Build history of the part. All positions in model axes, mm. Face numbers are marked on the shaded views. A direction names the side the tool comes from. Coordinates: 2 decimals unless noted, no trailing zeros. Loops run counter-clockwise (first coordinate to the right, second up) from the corner with the lowest first, then second, coordinate; pieces in that order, holes last. Notation, with made-up numbers: (-40, 29.25) - (9, 29.25) arc R16 ccw to (9, 58.25) - close; hole circle Ø9 at (-0.5, 83.5). An arc over 180 degrees is marked (long way). One line per item, written item: value.
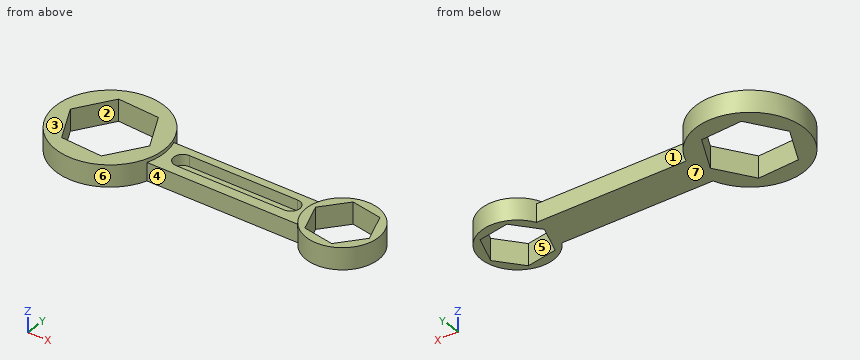
Autodesk Fusion 360 part; units mm, degrees
sketch "Sketch1" plane through (0, 0, 0) normal (0, 0, 1) x (1, 0, 0) in component "ex2"
  circle A0 centre (0, 0) radius 30
  circle A1 centre (129, 0) radius 20
  line L0 (12.7246, 19.2722) -> (-10.328, 20.6559)
  line L1 (-10.328, 20.6559) -> (-23.0525, 1.3837)
  line L2 (-23.0525, 1.3837) -> (-12.7246, -19.2722)
  line L3 (-12.7246, -19.2722) -> (10.328, -20.6559)
  line L4 (10.328, -20.6559) -> (23.0525, -1.3837)
  line L5 (23.0525, -1.3837) -> (12.7246, 19.2722)
  line L6 (146.0675, -2.9498) -> (140.0883, 13.306)
  line L7 (140.0883, 13.306) -> (123.0208, 16.2558)
  line L8 (123.0208, 16.2558) -> (111.9325, 2.9498)
  line L9 (111.9325, 2.9498) -> (117.9117, -13.306)
  line L10 (117.9117, -13.306) -> (134.9792, -16.2558)
  line L11 (134.9792, -16.2558) -> (146.0675, -2.9498)
  line L12 (28.4216, 9.6028) -> (111.4561, 9.6028)
  line L13 (28.1407, -10.3972) -> (111.915, -10.3972)
  line L14 (70.2554, 9.6028) -> (70.2554, -10.3972) construction
  line L15 (40.1843, 5.2583) -> (100.1843, 5.2583)
  line L16 (100.1843, -4.7417) -> (40.1843, -4.7417)
  arc A2 (40.1843, 5.2583) -> (40.1843, -4.7417) centre (40.1843, 0.2583) ccw
  arc A3 (100.1843, -4.7417) -> (100.1843, 5.2583) centre (100.1843, 0.2583) ccw
  point P0 (129, 0)
  dimension "d1" = 60
  dimension "d2" = 40
  dimension "d3" = 129
  dimension "d4" = 20
  dimension "d5" = 15
  dimension "d6" = 20
  dimension "d9" = 60
  dimension "d10" = 10
extrude "Extrude1" add sketch "Sketch1" along normal blind 10 contours A0 A1 L12 L13 in component "ex2"
sketch "Sketch1 (2)" plane through (0, 0, 0) normal (0, 0, 1) x (1, 0, 0)
  line L0 (30, 0) -> (46.6152, 0) construction
sketch "Sketch2" plane through (0, 0, 0) normal (0, 0, 1) x (1, 0, 0)
  line L0 (40, 5) -> (100, 5)
  line L1 (100, -5) -> (40, -5)
  arc A0 (40, 5) -> (40, -5) centre (40, 0) ccw
  arc A1 (100, -5) -> (100, 5) centre (100, 0) ccw
  dimension "d7" = 10
  dimension "d8" = 60
sketch "Sketch2 (2)" plane through (0, 0, 0) normal (0, 0, 1) x (1, 0, 0) in component "ex2"
extrude "Extrude2" add sketch "Sketch1" along normal blind 12 contours A0 | A1 in component "ex2"
extrude "Extrude3" add sketch "Sketch1" along normal blind 4 contours L15 L16 A2 A3 in component "ex2"
component "ex2" placed x (1, 0, 0) y (0, 1, 0) z (0, 0, 1) at (0, 0, 0)
Item 1: Cut at C-C, the plane z = 6.25. Write the cut outline in (x, y) (1 decimal), then the cut area to 3 significant figures.
Check result:
outline: (28.1, -10.4) - (111.9, -10.4) arc R20 ccw (long way) to (111.5, 9.6) - (28.4, 9.6) arc R30 ccw (long way) to start; hole (-23.1, 1.4) - (-12.7, -19.3) - (10.3, -20.7) - (23.1, -1.4) - (12.7, 19.3) - (-10.3, 20.7) - close; hole (40.2, -4.7) - (100.2, -4.7) arc R5 ccw to (100.2, 5.3) - (40.2, 5.3) arc R5 ccw to start; hole (111.9, 2.9) - (117.9, -13.3) - (135, -16.3) - (146.1, -2.9) - (140.1, 13.3) - (123, 16.3) - close
area: 2,850 mm^2
Item 2: Cut at D-D, the plane x = 0. Write the cut outline in (y, z).
Check result:
outline: (-30, 0) - (-20.04, 0) - (-20.04, 12) - (-30, 12) - close; (20.04, 0) - (30, 0) - (30, 12) - (20.04, 12) - close
Item 3: Pull direction Y, two halves, no side cores. Call the marked faces 5, 6 and 7: released by +Y, released by -Y, zero draft, split by the parting line, or undercut.
Check result:
face 5: undercut
face 6: split by the parting line
face 7: zero draft
Item 4: Cut at B-B, the plane x = 49.5. Write the cut outline in (y, z), then the cut area to 3 significant figures.
Check result:
outline: (-10.4, 0) - (9.6, 0) - (9.6, 10) - (5.26, 10) - (5.26, 4) - (-4.74, 4) - (-4.74, 10) - (-10.4, 10) - close
area: 140 mm^2
Item 5: Cut at A-A, the plane x = 129. Write the cut outline in (y, z), then the cut area to 3 significant figures.
Check result:
outline: (-20, 0) - (-15.22, 0) - (-15.22, 12) - (-20, 12) - close; (15.22, 0) - (20, 0) - (20, 12) - (15.22, 12) - close
area: 115 mm^2
Item 6: Drop flat-ended pins along their axis: P1, Ø16, axis at x = 86, y = -2, coming from the +Z side; P2, Ø5, axis at x = 87, y = -0.5, coming from the +Z side; P3, Ø4, axis at x = 47.5, z = 6.5, coming from the +Y side. Give the stop position or say it passes through.
Check result:
P1: stops at z = 10
P2: stops at z = 4
P3: stops at y = 9.6
Item 7: Tool access for the marked faces 1, 2, 3 and 4: list every direction of +Z, -Z, +X, -X, +Y, -Y with a clear straight run to the whole face (end or side of a thin tool).
Check result:
face 1: +Z, -Z, +Y
face 2: +Z, -Z
face 3: +Z, +X, -X, +Y, -Y
face 4: +Z, -Z, -Y
Item 8: Probe probe 1 along X at (y, z) = (-2, 7); probe 2 along X at (y, z) = (-3.5, 6.75); probe 3 along X at (y, z) = (-5, 6). List the from-to ranges inside material, lowest first. Write a range as from..to.
Check result:
probe 1: x = -29.93..-21.36, 22.65..35.72, 104.65..113.75, 145.72..148.9
probe 2: x = -29.8..-20.61, 21.66..36.89, 103.48..114.3, 145.61..148.69
probe 3: x = -29.58..-19.86, 20.66..114.86, 144.36..148.36
